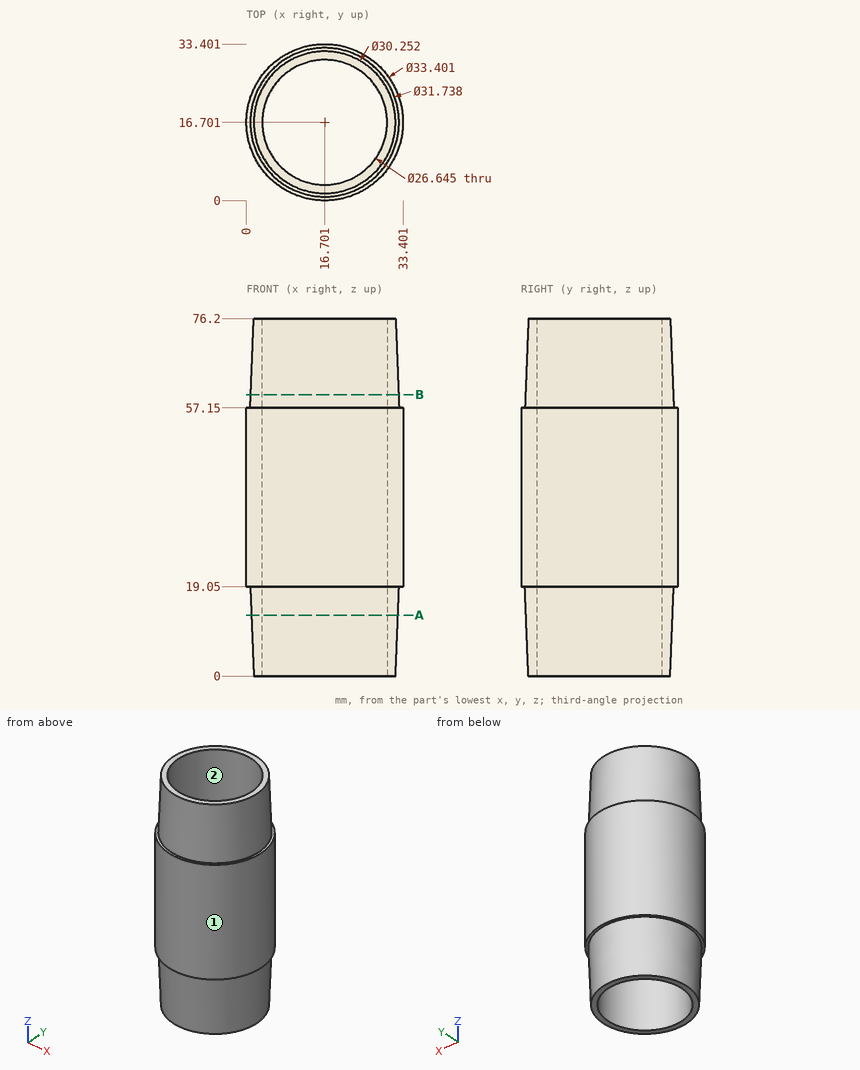
The drawing under review shows one solid part. Ordinate dimensions are in mm from its lowest x, y, z. Give positions to 0.01 mm unless a question says otherwise; leave off trailing zeros. Write each loop counter-clockwise with the first axis right and the second up, starting at its lowest first coordinate (ties: lowest second). Pieces come first, ordered by that corner, then holes. Notation, with made-up numbers: (43, 83) - (72, 83) arc R20 ccw to (72, 88) - close; hole circle Ø11 at (85, 83). An arc over 180 degrees is marked (long way). Answer in a Markdown table with one row per item. Add a question column.
1. Insertion check: P1, Ø1, axis at x = 27, z = 14, coming from the -Y side; P2, Ø12, axis at y = 27, z = 55.5, coming from the +X side; P3, Ø8, axis at x = 11.5, z = 61, coming from the -Y side (1 decimal); P4, Ø10, axis at x = 22, y = 14, coming from the -Z side. Each pin has a flat end and moves straight along its axis. Give the tip position at first contact, or say it passes through.
2. We need section A-A on z = 13. Write out the cut boundary in (x, y) (1 decimal), then the cut area to 3 significant figures.
3. Draft analysis for pull direction Y (two halves, no side actions). For the marked faces 1 and 2, state which applies: +Y half, -Y half, draft (parallel to the pull), parting line (faces both ways), or undercut.
4. We need section B-B on z = 60. Write out the cut boundary in (x, y) (1 decimal).
5. Wall thickness on line 1 along X through (y, z) = (28, 16) (1 decimal); line 2 along Z through (x, y) = (7.5, 30); line 3 along Y through (x, z) = (15, 63.5) (1 decimal): over which ranges is each line inside the solid? List them lowest first. Write a range as [from, to].
Ans:
| question | item | result |
|---|---|---|
| 1 | P1 | stops at y = 4.47 |
| 1 | P2 | stops at x = 32.84 |
| 1 | P3 | stops at y = 0.5 |
| 1 | P4 | passes through |
| 2 | outline | circle Ø31.3 at (16.7, 16.7); hole circle Ø26.6 at (16.7, 16.7) |
| 2 | area | 210 mm^2 |
| 3 | face 1 | parting line |
| 3 | face 2 | undercut |
| 4 | outline | circle Ø31.5 at (16.7, 16.7); hole circle Ø26.6 at (16.7, 16.7) |
| 5 | line 1 | x = [5.7, 9.6], [23.8, 27.7] |
| 5 | line 2 | z = [19.05, 57.15] |
| 5 | line 3 | y = [1.2, 3.5], [29.9, 32.2] |
